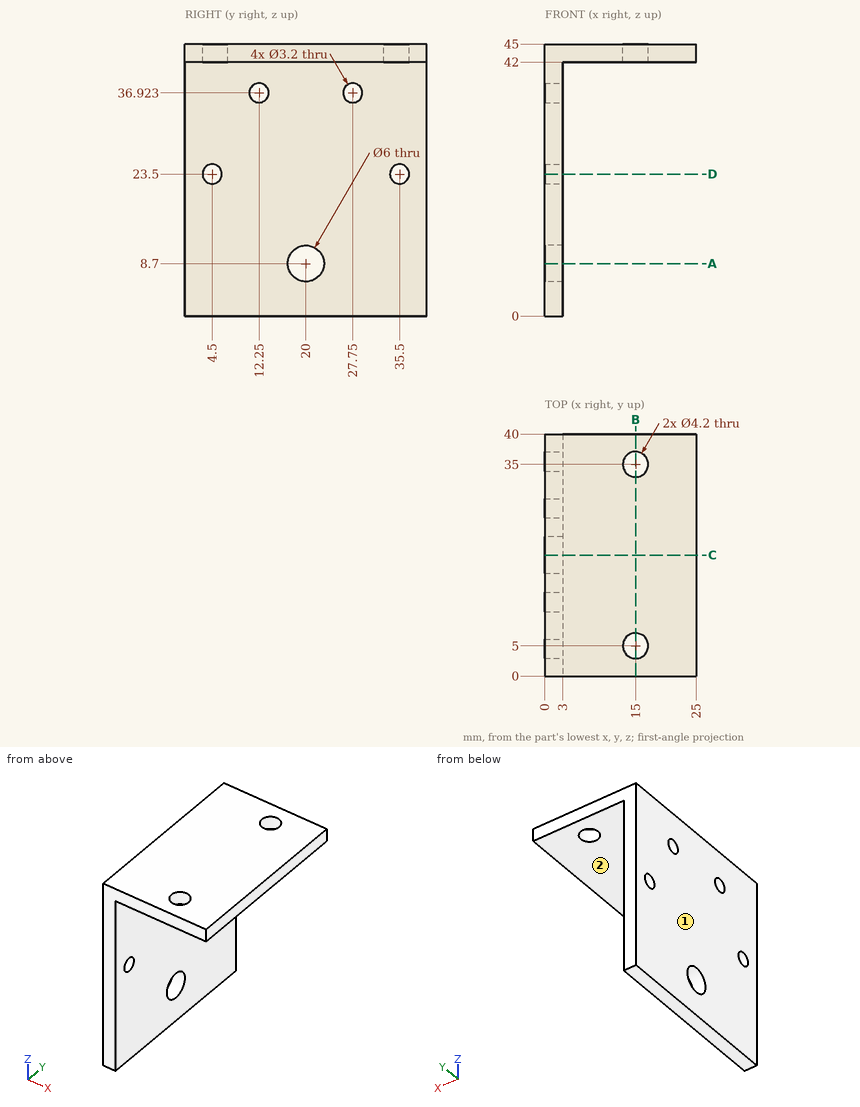
Geometry: see drawing. Coordinates: mm, zero at the bounding-box minimum. A direction names the side the tool comes from. Coordinates: 2 decimals unless noted, no trailing zeros. Loops run counter-clockwise (first coordinate to the right, second up) from the corner with the lowest first, then second, coordinate; pieces in that order, holes last. Notation, with made-up numbers: M 0,-38.75 L 32,-38.75 A23 cw 32,-18.75 Z; hole C -24.75,-12.5 d7. An arc over 180 degrees is marked long. Answer in a Markdown table with one row per item.
Q1. Section D-D on z = 23.5. Return the cut outline in (x, y).
Answers below:
| item | result |
|---|---|
| outline | M 0,0 L 3,0 L 3,2.9 L 0,2.9 Z; M 0,6.1 L 3,6.1 L 3,33.9 L 0,33.9 Z; M 0,37.1 L 3,37.1 L 3,40 L 0,40 Z |
Q2. Section C-C on y = 20. Return the cut outline in (x, z), plus the area to 3 significant figures.
Answers below:
| item | result |
|---|---|
| outline | M 0,0 L 3,0 L 3,5.7 L 0,5.7 Z; M 0,11.7 L 3,11.7 L 3,42 L 25,42 L 25,45 L 0,45 Z |
| area | 183 mm^2 |
Q3. First-contact query: pin 1 (6.5 mm diameter, centred on x = 16.5, y = 21, fed in from -Z); pin 2 (2.5 mm diameter, centred on y = 35.5, z = 23.5, fed in from -X); pin 3 (20 mm diameter, centred on y = 10.5, z = 22.5, fed in from +X). Flat tips, straight axial feed; report the tip coordinate or a pass-through.
Answers below:
| item | result |
|---|---|
| pin 1 | stops at z = 42 |
| pin 2 | passes through |
| pin 3 | stops at x = 3 |
Q4. Ray query, probe 1 along Z at (x, y) = (1.65, 20); probe 2 along Y at (x, z) = (2.5, 23); probe 3 along Z at (x, y) = (10, 15.5). Return the intervals inside material, ascending. Write a range as from..to.
Answers below:
| item | result |
|---|---|
| probe 1 | z = 0..5.7, 11.7..45 |
| probe 2 | y = 0..2.98, 6.02..33.98, 37.02..40 |
| probe 3 | z = 42..45 |
Q5. Section B-B on x = 15. Return the cut outline in (y, z).
Answers below:
| item | result |
|---|---|
| outline | M 0,42 L 2.9,42 L 2.9,45 L 0,45 Z; M 7.1,42 L 32.9,42 L 32.9,45 L 7.1,45 Z; M 37.1,42 L 40,42 L 40,45 L 37.1,45 Z |
Q6. Section A-A on z = 8.7. Return the cut outline in (x, y), plus the area to 3 significant figures.
Answers below:
| item | result |
|---|---|
| outline | M 0,0 L 3,0 L 3,17 L 0,17 Z; M 0,23 L 3,23 L 3,40 L 0,40 Z |
| area | 102 mm^2 |
Q7. Set-up query: the marked faces 1 and 2. Return all of +Z, -Z, +X, -X, +Y, -Y with unobstructed straight access to the full face (end or side cutting, diameter ignored); none if empty.
Answers below:
| item | result |
|---|---|
| face 1 | +Z, -Z, -X, +Y, -Y |
| face 2 | -Z, +X, +Y, -Y |
